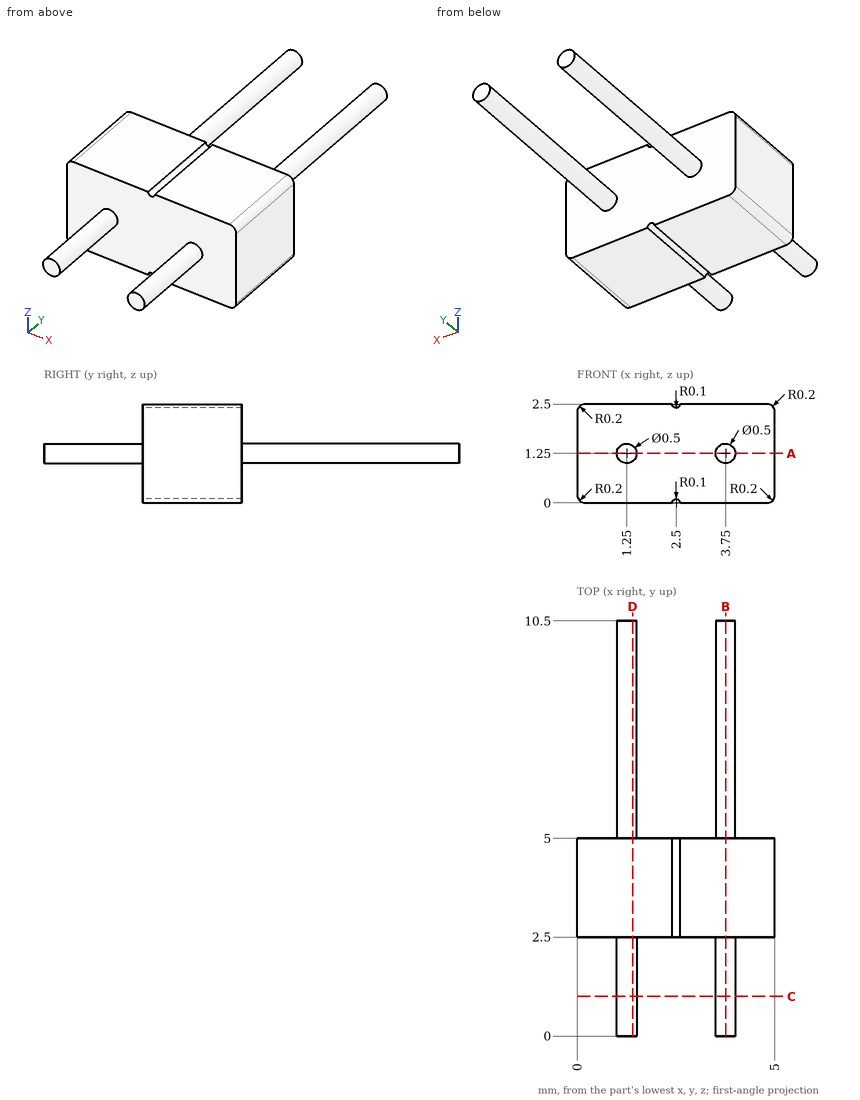
For this review, use the dimensioned drawing (mm, ordinates from the lowest corner) and the shaded views. Round coordinates to 2 decimals unless told otherwise and drop trailing zeros. Loops run counter-clockwise (first coordinate to the right, second up) from the corner with the lowest first, then second, coordinate; pieces in that order, holes last. Notation, with made-up numbers: M 10,31 L 46,31 A10 ccw 46,43 Z; hole C -31.5,-31.5 d6. An arc over 180 degrees is marked long. Answer as a JSON object with one key per item and string values.
(1) Take a section at A-A on z = 1.25. Give the boundary of the cut face in (x, y), and give its area (3 significant figures).
Resolved:
{"outline": "M 0,2.5 L 1,2.5 L 1,0 L 1.5,0 L 1.5,2.5 L 3.5,2.5 L 3.5,0 L 4,0 L 4,2.5 L 5,2.5 L 5,5 L 4,5 L 4,10.5 L 3.5,10.5 L 3.5,5 L 1.5,5 L 1.5,10.5 L 1,10.5 L 1,5 L 0,5 Z", "area": "20.5 mm²"}
(2) Take a section at C-C on y = 1. Give the boundary of the cut face in (x, z), and give its area (3 significant figures).
Resolved:
{"outline": "C 1.25,1.25 d0.5; C 3.75,1.25 d0.5", "area": "0.393 mm²"}
(3) Take a section at D-D on x = 1.4. Give the boundary of the cut face in (y, z), and give its area (3 significant figures).
Resolved:
{"outline": "M 0,1.05 L 2.5,1.05 L 2.5,0 L 5,0 L 5,1.05 L 10.5,1.05 L 10.5,1.45 L 5,1.45 L 5,2.5 L 2.5,2.5 L 2.5,1.45 L 0,1.45 Z", "area": "9.45 mm²"}
(4) To check wall thickness, follow line 1 along Y through (x, z) = (3.2, 0.55); line 2 along Z through (x, y) = (3.75, 9); line 3 along X through (y, z) = (8.5, 1.15). State the ranges of each line that lie inside material, in increasing order.
Resolved:
{"line 1": "2.5 to 5", "line 2": "1 to 1.5", "line 3": "1.02 to 1.48, 3.52 to 3.98"}
(5) Clearance check with a flat-ended pin moving along its axis: P1, Ø1.5, axis at x = 3.5, y = 7, coming from the -Z side. State where the tip first meets the part, or that it passes through.
Resolved:
{"P1": "z = 1"}
(6) Take a section at B-B on x = 3.75. Give the boundary of the cut face in (y, z).
Resolved:
{"outline": "M 0,1 L 2.5,1 L 2.5,0 L 5,0 L 5,1 L 10.5,1 L 10.5,1.5 L 5,1.5 L 5,2.5 L 2.5,2.5 L 2.5,1.5 L 0,1.5 Z"}
